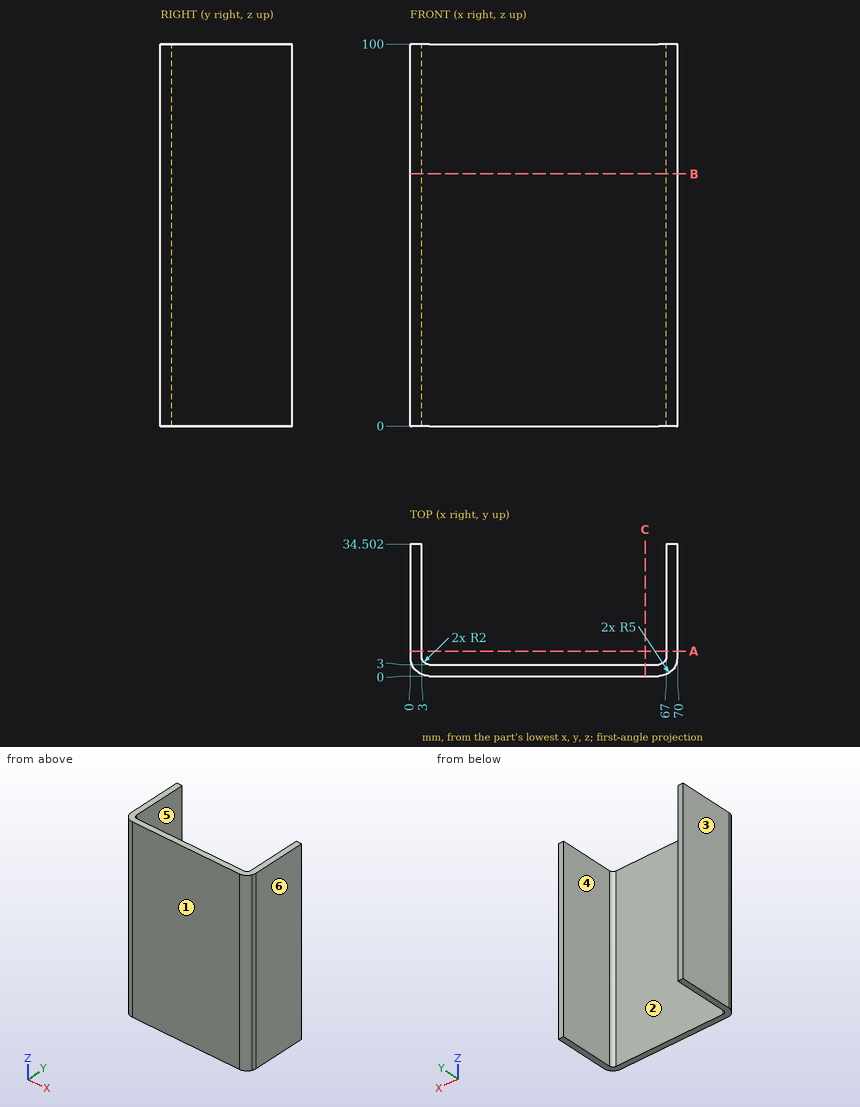
For this review, use the dimensioned drawing (mm, ordinates from the lowest corner) and the shaded views. A direction names the side the tool comes from. Give positions to 0.01 mm unless a question says otherwise; leave off trailing zeros. Order: outer loops, then holes, each group sorted by start corner. A loop starts at its lowest first (then second) coordinate and runs counter-clockwise, first axis right, second up.
1. Add section B-B, the plane z = 66. State the section outline as (x, y) points, then the cut area to 3 significant figures.
Solution:
outline: (0, 5) arc R5 ccw to (5, 0) - (65, 0) arc R5 ccw to (70, 5) - (70, 34.5) - (67, 34.5) - (67, 5) arc R2 cw to (65, 3) - (5, 3) arc R2 cw to (3, 5) - (3, 34.5) - (0, 34.5) - close
area: 390 mm2
2. Add section A-A, the plane y = 6.5. State the section outline as (x, z) points, then the cut area to 3 significant figures.
Solution:
outline: (0, 0) - (3, 0) - (3, 100) - (0, 100) - close; (67, 0) - (70, 0) - (70, 100) - (67, 100) - close
area: 600 mm2
3. Add section C-C, the plane x = 61.5. State the section outline as (y, z) points, then the cut area to 3 significant figures.
Solution:
outline: (0, 0) - (3, 0) - (3, 100) - (0, 100) - close
area: 300 mm2
4. To check wall thickness, follow L1, parallel to X at y = 32.5, z = 24; L2, parallel to Y at x = 53.5, z = 72; L3, parallel to Y at x = 65.5, z = 14.5 (1 decimal). State the ranges of each line that lie inside material, in increasing order.
Solution:
L1: x = 0 to 3, 67 to 70
L2: y = 0 to 3
L3: y = 0 to 3.1
5. Mouldability with a two-part tool opening along X and no side actions: class the marked faces 1, 2, 3 and 4 as +X half, -X half, draft (parallel to the pull), parting line (faces both ways), or undercut.
Solution:
face 1: draft
face 2: undercut
face 3: -X half
face 4: undercut
6. Tool access review of the marked faces 5 and 6: name each direction out of +Z, -Z, +X, -X, +Y, -Y from which nothing blocks a thin tool from reaching the whole face with its end or side.
Solution:
face 5: +Z, -Z, +Y
face 6: +Z, -Z, +X, +Y, -Y
